```python
from build123d import *

# Parameters (mm, degrees)
SKETCH_1_W          = 200
SKETCH_1_H          = 54
SKETCH_1_R          = 2.1
EXTRUDE_1_DEPTH     = 3
SKETCH_3_W          = 200
SKETCH_3_H          = 14
EXTRUDE_2_DEPTH     = 3
SKETCH_2_R          = 1.6
CUT_EXTRUDE_1_DEPTH = 10
SKETCH_7_W          = 15
SKETCH_7_H          = 68
CUT_EXTRUDE_3_DEPTH = 10
SKETCH_8_W          = 185
SKETCH_8_H          = 3
EXTRUDE_3_DEPTH     = 3
SKETCH_9_R          = 1.6
CUT_EXTRUDE_4_DEPTH = 10
SKETCH_10_W         = 35
SKETCH_10_H         = 71
EXTRUDE_4_DEPTH     = 3
SKETCH_12_W         = 26.5
SKETCH_12_H         = 42
CUT_EXTRUDE_6_DEPTH = 10
FILLET_1_R          = 15
FILLET_2_R          = 2


with BuildPart() as part:
    # 草图1 → 凸台-拉伸1 (new body)
    with BuildSketch(Plane.XY):
        Rectangle(SKETCH_1_W, SKETCH_1_H)
        with Locations((-47.5, 21)):
            Circle(SKETCH_1_R, mode=Mode.SUBTRACT)
        with Locations((-47.5, 4)):
            Circle(SKETCH_1_R, mode=Mode.SUBTRACT)
        with Locations((-47.5, -21)):
            Circle(SKETCH_1_R, mode=Mode.SUBTRACT)
        with Locations(Location((47.5, -21, 0), (0, 0, 180))):
            Circle(SKETCH_1_R, mode=Mode.SUBTRACT)
        with Locations(Location((47.5, 4, 0), (0, 0, 180))):
            Circle(SKETCH_1_R, mode=Mode.SUBTRACT)
        with Locations(Location((47.5, 21, 0), (0, 0, 180))):
            Circle(SKETCH_1_R, mode=Mode.SUBTRACT)
    extrude(amount=EXTRUDE_1_DEPTH)

    # 草图3 → 凸台-拉伸2 (add)
    with BuildSketch(Plane.XY.offset(3)):
        with Locations((0, -34)):
            Rectangle(SKETCH_3_W, SKETCH_3_H)
    extrude(amount=-EXTRUDE_2_DEPTH)

    # 草图2 → 切除-拉伸1 (cut)
    with BuildSketch(Plane.XY.offset(3)):
        with Locations((59, 9.5)):
            Circle(SKETCH_2_R)
        with Locations((81, 9.5)):
            Circle(SKETCH_2_R)
        with Locations((81, -35.5)):
            Circle(SKETCH_2_R)
        with Locations((59, -35.5)):
            Circle(SKETCH_2_R)
    extrude(amount=-CUT_EXTRUDE_1_DEPTH, mode=Mode.SUBTRACT)

    # 草图7 → 切除-拉伸3 (cut)
    with BuildSketch(Plane.XY.offset(3)):
        with Locations((92.5, -7)):
            Rectangle(SKETCH_7_W, SKETCH_7_H)
    extrude(amount=-CUT_EXTRUDE_3_DEPTH, mode=Mode.SUBTRACT)

    # 草图8 → 凸台-拉伸3 (add)
    with BuildSketch(Plane.XY.offset(3)):
        with Locations((-7.5, 28.5)):
            Rectangle(SKETCH_8_W, SKETCH_8_H)
    extrude(amount=-EXTRUDE_3_DEPTH)

    # 草图9 → 切除-拉伸4 (cut)
    with BuildSketch(Plane.XY.offset(3)):
        with Locations((-12.5, 26)):
            Circle(SKETCH_9_R)
        with Locations((7.5, 26)):
            Circle(SKETCH_9_R)
    extrude(amount=-CUT_EXTRUDE_4_DEPTH, mode=Mode.SUBTRACT)

    # 草图10 → 凸台-拉伸4 (add)
    with BuildSketch(Plane.XY.offset(3)):
        with Locations((102.5, -5.5)):
            Rectangle(SKETCH_10_W, SKETCH_10_H)
    extrude(amount=-EXTRUDE_4_DEPTH)

    # 草图12 → 切除-拉伸6 (cut)
    with BuildSketch(Plane.XY.offset(3)):
        with Locations((106.75, -10.45)):
            Rectangle(SKETCH_12_W, SKETCH_12_H)
    extrude(amount=-CUT_EXTRUDE_6_DEPTH, mode=Mode.SUBTRACT)

    # 圆角1
    fillet_1_edges = [part.edges().sort_by_distance(p)[0] for p in [
        (93.5, -31.45, 1.5),
        (93.5, 10.55, 1.5),
    ]]
    fillet(fillet_1_edges, radius=FILLET_1_R)

    # 圆角2
    fillet_2_edges = [part.edges().sort_by_distance(p)[0] for p in [
        (120, 30, 1.5),
        (120, -41, 1.5),
        (120, 10.55, 1.5),
        (120, -31.45, 1.5),
        (-100, -41, 1.5),
        (-100, 30, 1.5),
    ]]
    fillet(fillet_2_edges, radius=FILLET_2_R)


solid = part.part
```
Input: part model. Units: mm. Frame: model coordinates. A direction names the side the tool comes from. Give positions to 0.01 mm unless a question says otherwise; leave off trailing zeros. Order: outer loops, then holes, each group sorted by start corner. A loop starts at its lowest first (then second) coordinate and runs counter-clockwise, first axis right, second up. Notation, with made-up numbers: M 79.5,72.5 L 112.5,72.5 A27 ccw 112.5,108.5 Z; hole C -29.75,32 d4. An arc over 180 degrees is marked long. Return JSON: item names as keys, results as strings.
Item 1: Cut plane B-B (y = 21). Return loops of the section in (x, z), then the cut area to 3 significant figures.
Solutions:
{"outline": "M -100,0 L -49.6,0 L -49.6,3 L -100,3 Z; M -45.4,0 L 45.4,0 L 45.4,3 L -45.4,3 Z; M 49.6,0 L 120,0 L 120,3 L 49.6,3 Z", "area": "635 mm^2"}
Item 2: Pull-direction query (Y, two-part tool) for faces 3 (the cylindrical face through (45.56, 4.8, 1.48)), 4 (the flat face through (8, -5, 0)); classes: +Y half, -Y half, draft (parallel to the pull), parting line (faces both ways), or undercut.
Solutions:
{"face 3": "undercut", "face 4": "draft"}
Item 3: Cut plane D-D (y = -21). Return loops of the section in (x, z).
Solutions:
{"outline": "M -100,0 L -49.6,0 L -49.6,3 L -100,3 Z; M -45.4,0 L 45.4,0 L 45.4,3 L -45.4,3 Z; M 49.6,0 L 94.21,0 L 94.21,3 L 49.6,3 Z"}
Item 4: Cut plane A-A (x = 47.5). Return loops of the section in (y, z).
Solutions:
{"outline": "M -41,0 L -23.1,0 L -23.1,3 L -41,3 Z; M -18.9,0 L 1.9,0 L 1.9,3 L -18.9,3 Z; M 6.1,0 L 18.9,0 L 18.9,3 L 6.1,3 Z; M 23.1,0 L 30,0 L 30,3 L 23.1,3 Z"}
Item 5: First-contact query: P1, Ø3.5, axis at x = -12.5, y = 26, coming from the -Z side. Flat tip, straight axial feed; report the tip coordinate or a pass-through.
Solutions:
{"P1": "z = 0"}
Item 6: Ray query, probe 1 along Y at (x, z) = (47.5, 2.3); probe 2 along X at (y, z) = (4.5, 2.75); probe 3 along X at (y, z) = (3, 0.9). Return the intervals inside material, ascending.
Solutions:
{"probe 1": "-41 to -23.1, -18.9 to 1.9, 6.1 to 18.9, 23.1 to 30", "probe 2": "-100 to -49.54, -45.46 to 45.46, 49.54 to 96.46", "probe 3": "-100 to -49.35, -45.65 to 45.65, 49.35 to 95.48"}
Item 7: Cut plane C-C (z = 1). State how many separate pieces and enclosed holes the cut face has, then the cut area to 3 significant figures.
Solutions:
{"separate pieces": "1", "enclosed holes": "12", "area": "14,500 mm^2"}
Item 8: Access query for faces 1 (the cylindrical face through (-46.37, -19.23, 1.48)), 2 (the cylindrical face through (98.01, 6.27, 1.48)). Directions: +Z, -Z, +X, -X, +Y, -Y. A direction counts if a zero-diameter tool reaches every point of the face in a straight line with its end or side. Return the directions, or none.
Solutions:
{"face 1": "+Z, -Z", "face 2": "+Z, -Z, +X"}
